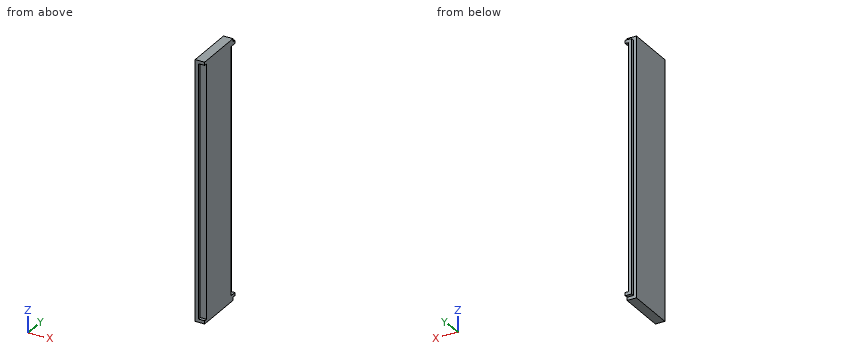
from build123d import *

# Parameters (mm, degrees)
EXTRUDE_1_DEPTH     = 820
SKETCH_2_W          = 10
SKETCH_2_H          = 10
EXTRUDE_2_DEPTH     = 20
SKETCH_4_W          = 20
SKETCH_4_H          = 20
EXTRUDE_3_DEPTH     = 10
SKETCH_5_W          = 10
SKETCH_5_H          = 10
CUT_EXTRUDE_2_DEPTH = 837.973715238


with BuildPart() as part:
    # Эскиз1 → Бобышка-Вытянуть1 (new body)
    with BuildSketch(Plane.XY):
        Polygon((0, 0), (0, 155), (10, 155), (10, 165), (20, 165), (20, 145), (30, 145), (30, 10), (10, 10), (10, 0), align=None)
    extrude(amount=EXTRUDE_1_DEPTH)

    # Эскиз2 → Бобышка-Вытянуть2 (add)
    with BuildSketch(Plane(origin=(10, 0, 0), x_dir=(0, 0, -1), z_dir=(1, 0, 0))):
        with Locations((-815, 5)):
            Rectangle(SKETCH_2_W, SKETCH_2_H)
        with Locations((-5, 5)):
            Rectangle(SKETCH_2_W, SKETCH_2_H)
    extrude(amount=EXTRUDE_2_DEPTH)

    # Эскиз4 → Бобышка-Вытянуть3 (add)
    with BuildSketch(Plane(origin=(20, 0, 0), x_dir=(0, 0, -1), z_dir=(1, 0, 0))):
        with Locations((-810, 155)):
            Rectangle(SKETCH_4_W, SKETCH_4_H)
        with Locations((-10, 155)):
            Rectangle(SKETCH_4_W, SKETCH_4_H)
    extrude(amount=EXTRUDE_3_DEPTH)

    # Эскиз5 → Вырез-Вытянуть2 (cut, through all)
    with BuildSketch(Plane(origin=(30, 0, 0), x_dir=(0, 0, -1), z_dir=(1, 0, 0))):
        with Locations((-815, 160)):
            Rectangle(SKETCH_5_W, SKETCH_5_H)
        with Locations((-5, 160)):
            Rectangle(SKETCH_5_W, SKETCH_5_H)
    extrude(amount=-CUT_EXTRUDE_2_DEPTH, mode=Mode.SUBTRACT)


solid = part.part
Geometry check sheet. Reference: the model listing, model coordinates, mm. Give positions to 0.01 mm unless a question says otherwise; leave off trailing zeros. Write each loop counter-clockwise with the first axis right and the second up, starting at its lowest first coordinate (ties: lowest second). Pieces come first, ordered by that corner, then holes. Notation, with made-up numbers: M -23.75,86 L 29.25,86 A26 cw 29.25,121 Z; hole C 88.25,49 d4. An arc over 180 degrees is marked long. Answer as CSV lines item,"result". Start each with the question number.
Q1. Section check B-B, the plane z = 265. Record the cut outline in (x, y), then the cut area to 3 significant figures.
Q2. Material ranges on L1, parallel to Z at x = 11.25, y = 9; L2, parallel to Y at x = 7.75, z = 230; L3, parallel to Y at x = 14.5, z = 624, recorded low to high.
Q3. Section check A-A, the plane x = 15.5. Record the cut outline in (y, z), then the cut area to 3 significant figures.
Q4. Go/stop test with flat-tipped pins: pin 1 (6 mm diameter, centred on y = 153.5, z = 567, fed in from +X); pin 2 (10 mm diameter, centred on x = 17.5, z = 450.5, fed in from -Y); pin 3 (12 mm diameter, centred on x = 5, z = 480, fed in from -Y); pin 4 (1 mm diameter, centred on x = 4, z = 410, fed in from +Y). Record where each tip stops, or that it passes through.
Geometry says:
1,outline,"M 0,0 L 10,0 L 10,10 L 30,10 L 30,145 L 20,145 L 20,165 L 10,165 L 10,155 L 0,155 Z"
1,area,"4,450 mm^2"
2,L1,"0 to 10, 810 to 820"
2,L2,"0 to 155"
2,L3,"10 to 165"
3,outline,"M 0,0 L 155,0 L 155,10 L 165,10 L 165,810 L 155,810 L 155,820 L 0,820 L 0,810 L 10,810 L 10,10 L 0,10 Z"
3,area,"127,000 mm^2"
4,pin 1,"x = 20"
4,pin 2,"y = 10"
4,pin 3,"y = 0"
4,pin 4,"y = 155"
